```python
from build123d import *

# Parameters (mm, degrees)
SKETCH1_R               = 5
SKETCH1_R_2             = 4
BOSS_EXTRUDE1_DEPTH     = 140
CUT_EXTRUDE1_DEPTH      = 175
CUT_EXTRUDE1_DEPTH_BACK = 175
SKETCH3_R               = 1.5
CUT_EXTRUDE2_DEPTH      = 10
CUT_EXTRUDE2_DEPTH_BACK = 10
SKETCH4_R               = 1.5


with BuildPart() as part:
    # Sketch1 → Boss-Extrude1 (new body)
    with BuildSketch(Plane.XY):
        Circle(SKETCH1_R)
        Circle(SKETCH1_R_2, mode=Mode.SUBTRACT)
    extrude(amount=BOSS_EXTRUDE1_DEPTH)

    # Sketch3 → Cut-Extrude1 (cut, two sides: drawn at the far end of the back side and taken through both)
    with BuildSketch(Plane(origin=(0, 0, 0), x_dir=(1, 0, 0), z_dir=(0, 1, 0)).offset(-CUT_EXTRUDE1_DEPTH_BACK)):
        with Locations(Location((0, -7.5, 0), (0, 0, 90))):
            Circle(SKETCH3_R)
    extrude(amount=CUT_EXTRUDE1_DEPTH + CUT_EXTRUDE1_DEPTH_BACK, mode=Mode.SUBTRACT)

    # Sketch4 → Cut-Extrude2 (cut, two sides: drawn at the far end of the back side and taken through both)
    with BuildSketch(Plane(origin=(0, 0, 0), x_dir=(1, 0, 0), z_dir=(0, 1, 0)).offset(-CUT_EXTRUDE2_DEPTH_BACK)):
        with Locations(Location((0, -132.5, 0), (0, 0, 90))):
            Circle(SKETCH4_R)
    extrude(amount=CUT_EXTRUDE2_DEPTH + CUT_EXTRUDE2_DEPTH_BACK, mode=Mode.SUBTRACT)


solid = part.part
```
Part model, mm, in its own coordinate system. Round coordinates to 2 decimals unless told otherwise and drop trailing zeros. Loops run counter-clockwise (first coordinate to the right, second up) from the corner with the lowest first, then second, coordinate; pieces in that order, holes last.
Item 1: Drill centre lines: line 1 (Y direction, x = 0, z = 65.5); line 2 (Y direction, x = 1.5, z = 44.5); line 3 (X direction, y = -4.45, z = 7.5). Where is each one in solid material? Low to high.
Item 2: Cut at C-C, the plane z = 45. Give the cut face in (x, y).
Item 3: Cut at A-A, the plane y = 0. Give the cut face in (x, z).
Item 4: Cut at B-B, the plane z = 7.5. Give the cut face in (x, y).
Item 5: Mould opens along Z. For faces 1 (the face through (1.846, -3.549, 69.02)), 2 (the face through (1.33, -4.37, 6.81)) say: +Z half, -Z half, draft (parallel to the pull), parting line (faces both ways), or undercut.
Item 6: Drop flat-ended pins along their axis: P1, Ø2, axis at x = -2.5, z = 68, coming from the +Y side; P2, Ø2.5, axis at x = 0, z = 7.5, coming from the -Y side; P3, Ø5, axis at y = -3.5, z = 109.5, coming from the +X side; P4, Ø5, axis at x = -3.5, z = 110.5, coming from the -Y side. Give the stop position or say it passes through.
A:
1. line 1: y = -5 to -4, 4 to 5
1. line 2: y = -4.77 to -3.71, 3.71 to 4.77
1. line 3: x = -2.28 to -1.5, 1.5 to 2.28
2. outline: circle Ø10 at (0, 0); hole circle Ø8 at (0, 0)
3. outline: (-5, 0) - (-4, 0) - (-4, 140) - (-5, 140) - close; (4, 0) - (5, 0) - (5, 140) - (4, 140) - close
4. outline: (-1.5, -4.77) - (-1.5, -3.71) arc R4 cw to (-1.5, 3.71) - (-1.5, 4.77) arc R5 ccw to start; (1.5, -4.77) arc R5 ccw to (1.5, 4.77) - (1.5, 3.71) arc R4 cw to (1.5, -3.71) - close
5. face 1: draft
5. face 2: undercut
6. P1: stops at y = 4.77
6. P2: passes through
6. P3: stops at x = 4.9
6. P4: stops at y = -4.9
